Read the model definition and answer for the solid it produces. Units are mm, in the model's axes. A direction names the side the tool comes from. Coordinates: 2 decimals unless noted, no trailing zeros. Write each loop counter-clockwise with the first axis right and the second up, starting at its lowest first coordinate (ties: lowest second). Pieces come first, ordered by that corner, then holes. Notation, with made-up numbers: (81.5, 48) -> (102.5, 48) arc R26 ccw to (102.5, 68) -> close; hole circle Ø2 at (84, 66.5). An arc over 180 degrees is marked (long way). One line per item, written item: value. Start each with the question number.
from build123d import *

# Parameters (mm, degrees)
F0_R     = 1.1
F1_DEPTH = 3


with BuildPart() as f1:
    # F0 (on Top) → F1 (new body)
    with BuildSketch(Plane.XY):
        with BuildLine():
            Line((8.5, 0), (5, 0))
            Line((5, 0), (5, 3))
            Line((5, 3), (0, 3))
            Line((0, 3), (0, 0))
            Line((0, 0), (0, -33))
            ThreePointArc((0, -33), (10, -43), (20, -33))
            Line((20, -33), (20, 0))
            Line((20, 0), (20, 3))
            Line((20, 3), (15, 3))
            Line((15, 3), (15, 0))
            Line((15, 0), (11.5, 0))
            Line((11.5, 0), (11.5, -2))
            Line((11.5, -2), (13, -2))
            Line((13, -2), (13, -4.5))
            Line((13, -4.5), (11.5, -4.5))
            Line((11.5, -4.5), (11.5, -7.5))
            Line((11.5, -7.5), (10, -7.5))
            Line((10, -7.5), (8.5, -7.5))
            Line((8.5, -7.5), (8.5, -4.5))
            Line((8.5, -4.5), (7, -4.5))
            Line((7, -4.5), (7, -2))
            Line((7, -2), (8.5, -2))
            Line((8.5, -2), (8.5, 0))
        make_face()
        with Locations((10, -33)):
            Circle(F0_R, mode=Mode.SUBTRACT)
    extrude(amount=F1_DEPTH)


solid = f1.part
1. A cutting plane is placed at A-A on x = 10. Give the vertices of the cut face in (y, z).
2. A tool of negligible diameter and unlimited length cuts with its end or side. For faces 1 (the face through (11.5, -6, 1)), 2 (the face through (10, -43, 1)), 3 (the face through (8, -4.5, 1)), from which of +Z, -Z, +X, -X, +Y, -Y can it reach the whole face along a straight path? Write none if from no direction.
3. Find the intervals of material crossed by probe 1 along Y at (x, z) = (10, 2.1); probe 2 along X at (y, z) = (-6, 2.55); probe 3 along X at (y, z) = (-33.5, 1), in increasing order. Write a range as from..to.
4. A cutting plane is placed at B-B on z = 1.8. Give the vertices of the cut face in (x, y), then the cut area to 3 significant figures.
5. For a pull along Y with two mould halves and no side action, classify faces 4 (the face through (11.5, -1, 1)), 5 (the face through (10.59, -32.07, 1.48)), 6 (the face through (18, 3, 1)) as +Y half, -Y half, draft (parallel to the pull), parting line (faces both ways), or undercut.
6. A cutting plane is placed at C-C on y = -35. Give the vertices of the cut face in (x, z).
7. Given pin 1 (1.5 mm diameter, centred on x = 6.5, z = 1, fed in from +Y); pin 2 (2 mm diameter, centred on x = 10, y = -33, fed in from -Z); pin 3 (0.8 mm diameter, centred on x = 7.5, z = 2, fed in from -Y); pin 4 (1.5 mm diameter, centred on x = 9.5, z = 1, fed in from +Y), each flat-ended and moving along its own axis, determine where each tip first touches the part or whether it passes through.
Derived:
1. outline: (-43, 0) -> (-34.1, 0) -> (-34.1, 3) -> (-43, 3) -> close; (-31.9, 0) -> (-7.5, 0) -> (-7.5, 3) -> (-31.9, 3) -> close
2. face 1: +Z, -Z, +Y
2. face 2: +Z, -Z, -Y
2. face 3: +Z, -Z
3. probe 1: y = -43..-34.1, -31.9..-7.5
3. probe 2: x = 0..8.5, 11.5..20
3. probe 3: x = 0.01..9.02, 10.98..19.99
4. outline: (0, -33) arc R10 ccw to (20, -33) -> (20, 3) -> (15, 3) -> (15, 0) -> (11.5, 0) -> (11.5, -2) -> (13, -2) -> (13, -4.5) -> (11.5, -4.5) -> (11.5, -7.5) -> (8.5, -7.5) -> (8.5, -4.5) -> (7, -4.5) -> (7, -2) -> (8.5, -2) -> (8.5, 0) -> (5, 0) -> (5, 3) -> (0, 3) -> close; hole circle Ø2.2 at (10, -33)
4. area: 813 mm2
5. face 4: draft
5. face 5: undercut
5. face 6: +Y half
6. outline: (0.2, 0) -> (19.8, 0) -> (19.8, 3) -> (0.2, 3) -> close
7. pin 1: stops at y = 0
7. pin 2: passes through
7. pin 3: stops at y = -42.78
7. pin 4: stops at y = -7.5
